from build123d import *

# Parameters (mm, degrees)
SKETCH_W   = 120.3
SKETCH_H   = 40.2
SKETCH_R   = 3
SKETCH_R_2 = 1.02
PAD_DEPTH  = 3.2


with BuildPart() as part:
    # Sketch → Pad (new body)
    with BuildSketch(Plane.XY):
        Rectangle(SKETCH_W, SKETCH_H)
        with Locations((-43.15, -12.1)):
            Circle(SKETCH_R, mode=Mode.SUBTRACT)
        with Locations((-33.65, -12.1)):
            Circle(SKETCH_R, mode=Mode.SUBTRACT)
        with Locations((-24.15, -12.1)):
            Circle(SKETCH_R, mode=Mode.SUBTRACT)
        with Locations((-14.65, -12.1)):
            Circle(SKETCH_R, mode=Mode.SUBTRACT)
        with Locations((13.85, -12.1)):
            Circle(SKETCH_R, mode=Mode.SUBTRACT)
        with Locations((-5.15, -12.1)):
            Circle(SKETCH_R, mode=Mode.SUBTRACT)
        with Locations((4.35, -12.1)):
            Circle(SKETCH_R, mode=Mode.SUBTRACT)
        with Locations((23.35, -12.1)):
            Circle(SKETCH_R, mode=Mode.SUBTRACT)
        Circle(SKETCH_R_2, mode=Mode.SUBTRACT)
        with BuildLine():
            Line((36.85, -5.4), (30.85, -5.4))
            ThreePointArc((30.85, -5.4), (30.142893, -5.692893), (29.85, -6.4))
            Line((29.85, -6.4), (29.85, -12.4))
            ThreePointArc((29.85, -12.4), (30.142893, -13.107107), (30.85, -13.4))
            Line((30.85, -13.4), (36.85, -13.4))
            ThreePointArc((36.85, -13.4), (37.557107, -13.107107), (37.85, -12.4))
            Line((37.85, -12.4), (37.85, -6.4))
            ThreePointArc((37.85, -6.4), (37.557107, -5.692893), (36.85, -5.4))
        make_face(mode=Mode.SUBTRACT)
    extrude(amount=PAD_DEPTH)


solid = part.part
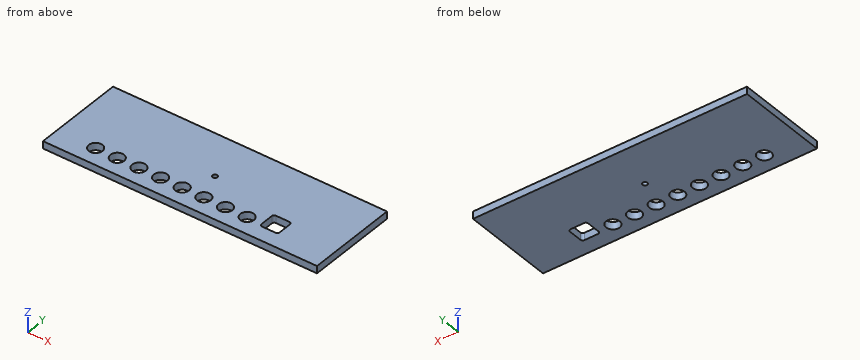
Can you work these out from the model? Positions are in its coordinate system, mm. Round coordinates to 2 decimals unless told otherwise and drop trailing zeros. Loops run counter-clockwise (first coordinate to the right, second up) from the corner with the lowest first, then second, coordinate; pieces in that order, holes last. Notation, with made-up numbers: (38, -3) - (80, -3) arc R21 cw to (80, 10) - close; hole circle Ø1 at (20.5, -1.5). An arc over 180 degrees is marked (long way). Use CSV: the item, a comma, the result in double quotes. Start each with the question number.
1) If we section it at C-C on z = 0.6: Count the separate pieces of the cut face and the enclosed holes in it, plus the area to 3 significant figures.
2) Please list where these lines run through material, in increasing order: probe 1 along Y at (x, z) = (23.35, 2.1); probe 2 along Y at (x, z) = (0, 1.5); probe 3 along X at (y, z) = (-8, 1.45). Write a range as [from, to].
3) If we section it at B-B on y = 0: Write out the boundary of the cut face in (x, z).
4) If we section it at A-A on x = 0: Write out the boundary of the cut face in (y, z), plus the area to 3 significant figures.
Geometry results:
1,separate pieces,"1"
1,enclosed holes,"10"
1,area,"4,540 mm2"
2,probe 1,"y = [-20.1, -15.1], [-9.1, 20.1]"
2,probe 2,"y = [-20.1, -1.02], [1.02, 20.1]"
2,probe 3,"x = [-60.15, 29.85], [37.85, 60.15]"
3,outline,"(-60.15, 0) - (-1.02, 0) - (-1.02, 3.2) - (-60.15, 3.2) - close; (1.02, 0) - (60.15, 0) - (60.15, 3.2) - (1.02, 3.2) - close"
4,outline,"(-20.1, 0) - (-1.02, 0) - (-1.02, 3.2) - (-20.1, 3.2) - close; (1.02, 0) - (20.1, 0) - (20.1, 3.2) - (1.02, 3.2) - close"
4,area,"122 mm2"
